Part print with two shaded views. Sizes in mm from the minimum x, y, z corner. A direction names the side the tool comes from. Coordinates: 2 decimals unless noted, no trailing zeros. Loops run counter-clockwise (first coordinate to the right, second up) from the corner with the lowest first, then second, coordinate; pieces in that order, holes last. Notation, with made-up numbers: (73, 1.5) -> (102, 1.5) arc R16 cw to (102, 18.5) -> close; hole circle Ø8 at (43, -8). An arc over 180 degrees is marked (long way). Return JSON: item names as keys, results as strings. Group by question number.
(1) Flat gauge pins, fed straight in: pin 1 Ø0.5 at (y, z) = (4, 10) entering from +X; pin 2 Ø0.5 at (x, z) = (8, 1) entering from +Y. Where does each tip first touch, or does it go through?
(2) Tool access for the marked faces 4, 5, 6, 7 and 8: list every direction of +Z, -Z, +X, -X, +Y, -Y with a clear straight run to the whole face (end or side of a thin tool).
(3) Saw through at B-B on x = 4. Write the cut outline in (y, z).
(4) Probe L1, parallel to Z at x = 4, y = 1.95; L2, parallel to X at y = 3.8, z = 0.5; L3, parallel to X at y = 1.35, z = 6. List the from-to ranges inside material, lowest first.
(5) Mould opens along Z. For the marked faces 1, 2 and 3 say: pulls with the +Z half, pulls with the -Z half, needs draft (parallel to the pull), parting line crosses it, or undercut.
(6) Saw through at D-D on z = 6. Write the cut outline in (x, y).
(7) Saw through at C-C on y = 1.15. Write the cut outline in (x, z) (1 decimal).
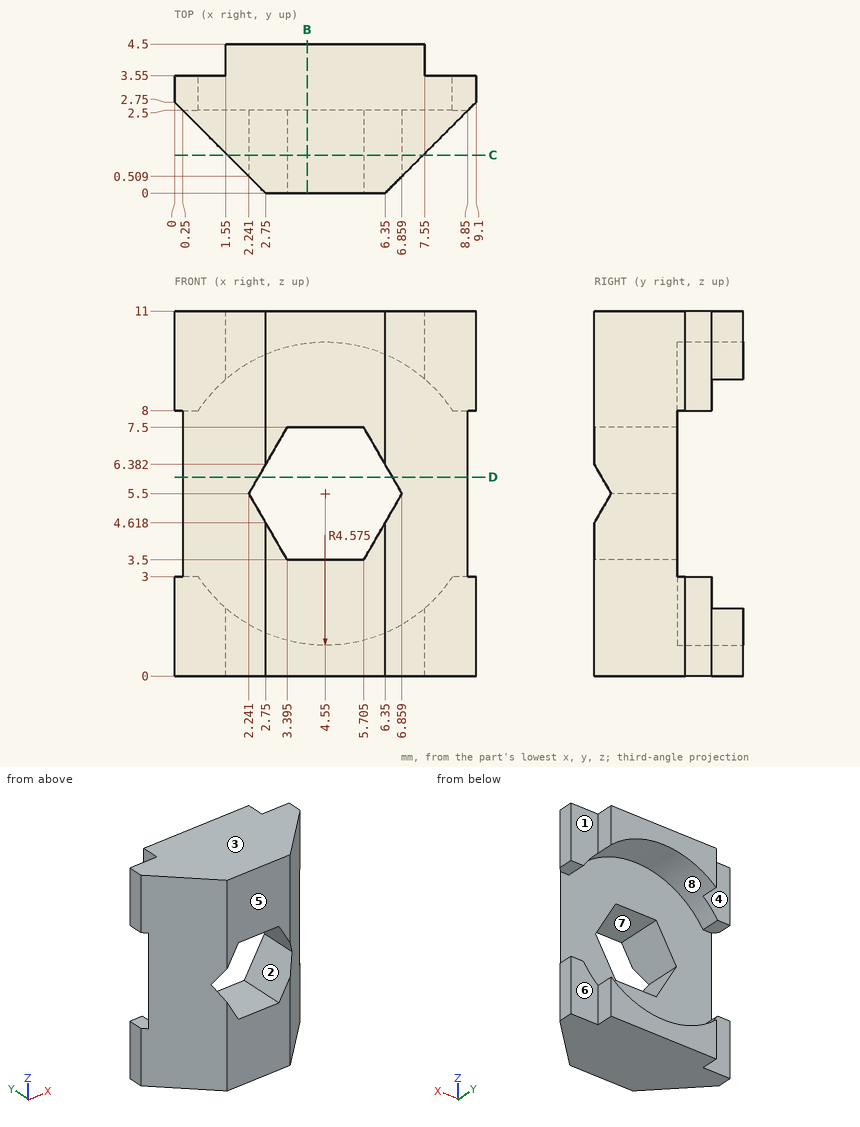
Geometry results:
{
 "1": {"pin 1": "x = 7.55", "pin 2": "y = 3.55"},
 "2": {"face 4": "+Z, -Z, -X, +Y", "face 5": "+Z, -Z, +X, -X, -Y", "face 6": "+Z, -Z, +X, +Y", "face 7": "+Y, -Y", "face 8": "+Y"},
 "3": {"outline": "(0, 0) -> (4.5, 0) -> (4.5, 0.96) -> (2.5, 0.96) -> (2.5, 3.5) -> (0, 3.5) -> close; (0, 7.5) -> (2.5, 7.5) -> (2.5, 10.04) -> (4.5, 10.04) -> (4.5, 11) -> (0, 11) -> close"},
 "4": {"L1": "0 to 3.5, 7.5 to 11", "L2": "1.55 to 7.55", "L3": "1.4 to 2.53, 6.57 to 7.7"},
 "5": {"face 1": "needs draft", "face 2": "undercut", "face 3": "pulls with the +Z half"},
 "6": {"outline": "(0.25, 2.5) -> (2.53, 0.22) -> (2.53, 2.5) -> close; (6.57, 0.22) -> (8.85, 2.5) -> (6.57, 2.5) -> close"},
 "7": {"outline": "(1.6, 0) -> (7.5, 0) -> (7.5, 11) -> (1.6, 11) -> close; hole (2.2, 5.5) -> (3.4, 3.5) -> (5.7, 3.5) -> (6.9, 5.5) -> (5.7, 7.5) -> (3.4, 7.5) -> close"}
}
